Work out the finished part from the listing and answer in its coordinate system (mm). A direction names the side the tool comes from. Coordinates: 2 decimals unless noted, no trailing zeros. Write each loop counter-clockwise with the first axis right and the second up, starting at its lowest first coordinate (ties: lowest second). Pieces come first, ordered by that corner, then holes. Notation, with made-up numbers: (-40, 32.25) - (-14, 32.25) arc R22 cw to (-14, 39.25) - close; hole circle Ø7 at (-24.75, 50). An arc over 180 degrees is marked (long way). Use a Markdown table: item, result. Add a question column.
(1) Given pin 1 Ø4.5 at (x, z) = (2, 4.5) entering from -Y; pin 2 Ø2.5 at (y, z) = (-5.5, -3) entering from -X; pin 3 Ø6 at (x, z) = (35.5, 0) entering from -Y, each flat-ended and moving along its own axis, determine where each tip first touches the part or whether it passes through.
(2) A tool of negligible diameter and unlimited length cuts with its end or side. For faces 1 (the face through (34, -8, -7)), 2 (the face through (50, -7, -2)), 3 (the face through (48.5, -4, 0)), 4 (the face through (0, -1, 0)), 5 (the face through (3, -2, 0)), from which of +Z, -Z, +X, -X, +Y, -Y can it reach the whole face along a straight path? Write none if from no direction.
(3) For a pull along Z with two mould halves and no side action, classify faces 6 (the face through (28, -6, 6)), 7 (the face through (25, 0, 0)), 8 (the face through (32, -4, -9)) as released by +Z, released by -Z, zero draft, split by the parting line, or undercut.
(4) The part is cut by section B-B, the plane z = -4.5. Give the vertices of the cut face in (x, y).
(5) Find the intervals of material crossed by line 1 (Z direction, x = 28, y = -6.5); line 2 (X direction, y = -6.75, z = 3.5); line 3 (Y direction, x = 29.5, z = -5.25), in increasing order. Write a range as from..to.
(6) The part is cut by section D-D, the plane z = 7. Give the vertices of the cut face in (x, y).
(7) The part is cut by section C-C, the plane y = -4.75. Give the vertices of the cut face in (x, z).
(8) The part is cut by section A-A, the plane x = 36. Give the vertices of the cut face in (y, z).
from build123d import *

# Parameters (mm, degrees)
EXTRUDE_1_DEPTH     = 9
CUT_EXTRUDE_1_DEPTH = 5
CUT_EXTRUDE_2_REACH = 54.889


with BuildPart() as part:
    # 草图1 → 凸台-拉伸1 (new, symmetric)
    with BuildSketch(Plane.XY):
        Polygon((0, 0), (51.5, 0), (51.5, -8), (15, -8), (5.5, -2), (0, -2), align=None)
    extrude(amount=EXTRUDE_1_DEPTH, both=True)

    # 草图2 → 切除-拉伸1 (cut)
    with BuildSketch(Plane.XZ.offset(8)):
        Polygon((15, -6), (48.5, -6), (48.5, 6), (15, 6), (5.5, 6), (3, 6), (3, -6), (5.5, -6), align=None)
    extrude(amount=-CUT_EXTRUDE_1_DEPTH, mode=Mode.SUBTRACT)

    # 草图3 → 切除-拉伸2 (cut, up to next)
    with BuildSketch(Plane(origin=(51.5, 0, 0), x_dir=(0, 0, -1), z_dir=(1, 0, 0)), mode=Mode.PRIVATE) as cut_extrude_2_sk1:
        with BuildLine():
            Line((2, -6.3), (2, -8))
            Line((2, -8), (-2, -8))
            Line((-2, -8), (-2, -6.3))
            ThreePointArc((-2, -6.3), (0, -4.3), (2, -6.3))
        make_face()
    cut_extrude_2_tool1 = extrude(cut_extrude_2_sk1.sketch, amount=-CUT_EXTRUDE_2_REACH, mode=Mode.PRIVATE) & part.part
    add(cut_extrude_2_tool1.solids().sort_by_distance((51.5, -6.334141, 0))[0], mode=Mode.SUBTRACT)


solid = part.part
Model answer:
| question | item | result |
|---|---|---|
| 1 | pin 1 | y = -2 |
| 1 | pin 2 | x = 48.5 |
| 1 | pin 3 | y = -3 |
| 2 | face 1 | +Z, -Z, +X, -X, -Y |
| 2 | face 2 | +X, -X, -Y |
| 2 | face 3 | -X, -Y |
| 2 | face 4 | +Z, -Z, -X, +Y, -Y |
| 2 | face 5 | +Z, -Z, -X, -Y |
| 3 | face 6 | undercut |
| 3 | face 7 | zero draft |
| 3 | face 8 | released by -Z |
| 4 | outline | (0, -2) - (5.5, -2) - (7.08, -3) - (48.5, -3) - (48.5, -8) - (51.5, -8) - (51.5, 0) - (0, 0) - close |
| 5 | line 1 | -9..-6, 6..9 |
| 5 | line 2 | 48.5..51.5 |
| 5 | line 3 | -3..0 |
| 6 | outline | (0, -2) - (5.5, -2) - (15, -8) - (51.5, -8) - (51.5, 0) - (0, 0) - close |
| 7 | outline | (9.85, -9) - (51.5, -9) - (51.5, -1.26) - (48.5, -1.26) - (48.5, -6) - (9.85, -6) - close; (9.85, 6) - (48.5, 6) - (48.5, 1.26) - (51.5, 1.26) - (51.5, 9) - (9.85, 9) - close |
| 8 | outline | (-8, -9) - (0, -9) - (0, 9) - (-8, 9) - (-8, 6) - (-3, 6) - (-3, -6) - (-8, -6) - close |
